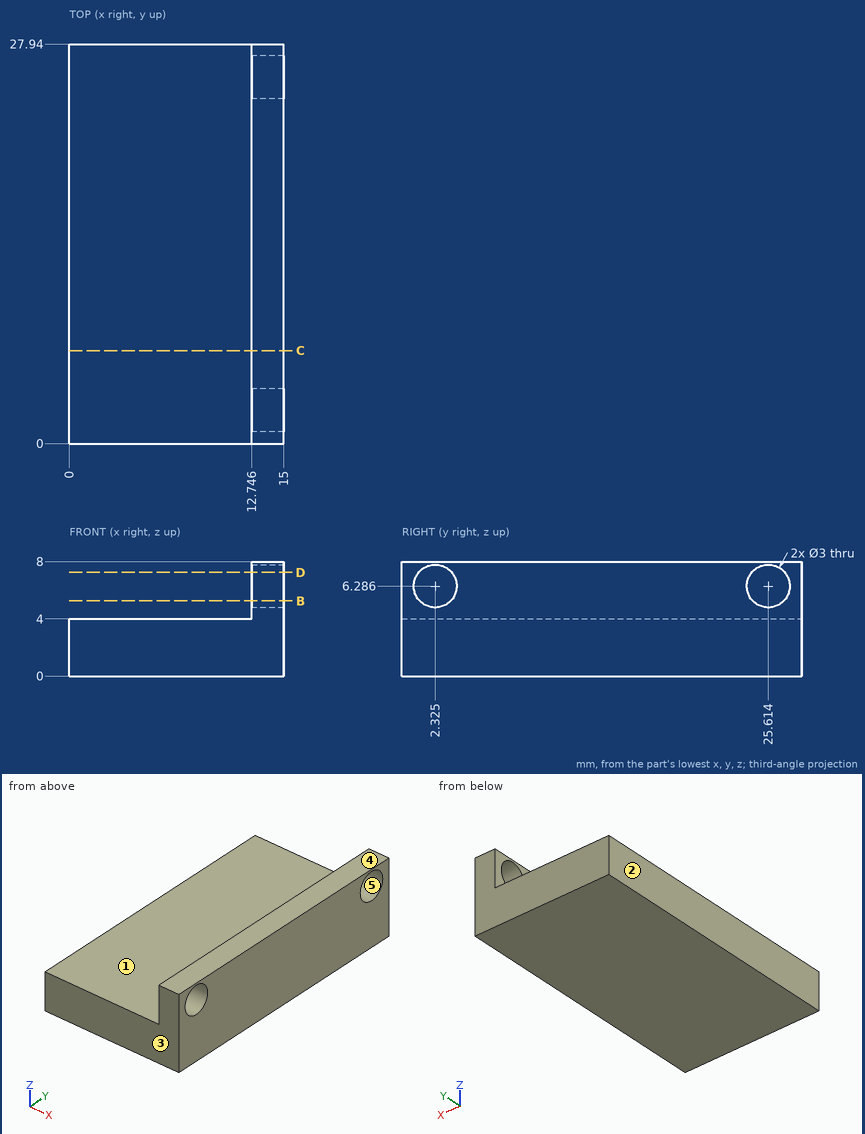
Print and shaded views of the part. All mm, measured from the part's lowest x, y and z. A direction names the side the tool comes from. Give positions to 0.01 mm unless a question says otherwise; leave off trailing zeros. Loops run counter-clockwise (first coordinate to the right, second up) from the corner with the lowest first, then second, coordinate; pieces in that order, holes last. Notation, with made-up numbers: (30.25, 30.5) -> (49.25, 30.5) arc R27 ccw to (49.25, 55.5) -> close; hole circle Ø6 at (83.5, 62). An arc over 180 degrees is marked (long way). One line per question, with ' | ' between items. Start each with the question number.
1) 3-axis set-ups, long thin cutter, end or side, ignore diameter. For the marked faces 1 and 2: which of +Z, -Z, +X, -X, +Y, -Y reach the whole face in a straight line?
2) Cut at D-D (z = 7.25). Give the cut face in (x, y) (1 decimal).
3) Pin check, flat tips, straight feed: pin 1 (4 mm diameter, centred on y = 3.5, z = 7, fed in from -X); pin 2 (2.5 mm diameter, centred on y = 2.325, z = 6.286, fed in from -X); pin 3 (4 mm diameter, centred on x = 9.5, y = 23, fed in from +Z). Stop position of each tip, or through.
4) Two-plate mould, pull along Z, no slides. Class the marked faces 3, 4 and 5: released by +Z, released by -Z, zero draft, split by the parting line, or undercut.
5) Cut at C-C (y = 6.5). Give the cut face in (x, z) (1 decimal).
6) Cut at B-B (z = 5.25). Give the cut face in (x, y) (1 decimal).
7) Probe L1, parallel to Z at x = 10, y = 7; L2, parallel to X at y = 16, z = 4.75 (1 decimal); L3, parallel to Z at x = 14.25, y = 24.5. List the from-to ranges inside material, lowest first.
Return value:
1) face 1: +Z, -X, +Y, -Y | face 2: +Z, -Z, -X, +Y, -Y
2) outline: (12.7, 0) -> (15, 0) -> (15, 1.2) -> (12.7, 1.2) -> close; (12.7, 3.5) -> (15, 3.5) -> (15, 24.5) -> (12.7, 24.5) -> close; (12.7, 26.8) -> (15, 26.8) -> (15, 27.9) -> (12.7, 27.9) -> close
3) pin 1: x = 12.75 | pin 2: through | pin 3: z = 4
4) face 3: zero draft | face 4: released by +Z | face 5: undercut
5) outline: (0, 0) -> (15, 0) -> (15, 8) -> (12.7, 8) -> (12.7, 4) -> (0, 4) -> close
6) outline: (12.7, 0) -> (15, 0) -> (15, 1.2) -> (12.7, 1.2) -> close; (12.7, 3.4) -> (15, 3.4) -> (15, 24.5) -> (12.7, 24.5) -> close; (12.7, 26.7) -> (15, 26.7) -> (15, 27.9) -> (12.7, 27.9) -> close
7) L1: 0 to 4 | L2: 12.7 to 15 | L3: 0 to 5.28, 7.29 to 8
